Geometry: final body of the model. Coordinates: model frame, mm. Face numbers are marked on the shaded views. A direction names the side the tool comes from. Coordinates: 2 decimals unless noted, no trailing zeros. Order: outer loops, then holes, each group sorted by start corner. A loop starts at its lowest first (then second) coordinate and runs counter-clockwise, first axis right, second up. Notation, with made-up numbers: M 68.5,42 L 95.5,42 A10 ccw 95.5,51 Z; hole C 12,66 d7. An arc over 180 degrees is marked long. One line per question, with ' | ' between items.
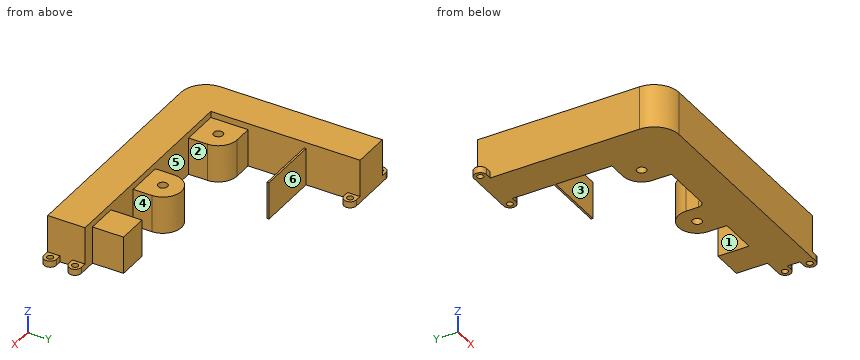
from build123d import *

# Parameters (mm, degrees)
F1_DEPTH = 70
F0_R     = 7.5
F0_W     = 100
F0_H     = 3
F0_W_2   = 50
F0_H_2   = 50
F2_DEPTH = 60
F0_R_2   = 5
F3_DEPTH = 10


with BuildPart() as f1:
    # F0 (on Top) → F1 (new body)
    with BuildSketch(Plane.XY):
        with BuildLine():
            Line((0, 280), (0, 40))
            ThreePointArc((0, 40), (11.715729, 11.715729), (40, 0))
            Line((40, 0), (400, 0))
            Line((400, 0), (400, 20))
            Line((400, 20), (400, 40))
            Line((400, 40), (400, 60))
            Line((400, 60), (380, 60))
            Line((380, 60), (330, 60))
            Line((330, 60), (270, 60))
            Line((270, 60), (210, 60))
            Line((210, 60), (200, 60))
            Line((200, 60), (120, 60))
            Line((120, 60), (60, 60))
            Line((60, 60), (60, 120))
            Line((60, 120), (60, 210))
            Line((60, 210), (60, 213))
            Line((60, 213), (60, 280))
            Line((60, 280), (60, 300))
            Line((60, 300), (0, 300))
            Line((0, 300), (0, 280))
        make_face()
    extrude(amount=F1_DEPTH)

    # F0 (on Top) → F2 (join)
    with BuildSketch(Plane.XY):
        with BuildLine():
            Line((90, 120), (60, 120))
            Line((60, 120), (60, 60))
            Line((60, 60), (120, 60))
            Line((120, 60), (120, 90))
            ThreePointArc((120, 90), (111.213203, 111.213203), (90, 120))
        make_face()
        with Locations((90, 90)):
            Circle(F0_R, mode=Mode.SUBTRACT)
        with BuildLine():
            Line((210, 60), (270, 60))
            Line((270, 60), (270, 90))
            ThreePointArc((270, 90), (240, 120), (210, 90))
            Line((210, 90), (210, 70))
            Line((210, 70), (210, 60))
        make_face()
        with Locations((240, 90)):
            Circle(F0_R, mode=Mode.SUBTRACT)
        with Locations((110, 211.5)):
            Rectangle(F0_W, F0_H)
        with Locations((355, 85)):
            Rectangle(F0_W_2, F0_H_2)
    extrude(amount=F2_DEPTH)

    # F0 (on Top) → F3 (join)
    with BuildSketch(Plane.XY):
        with BuildLine():
            Line((200, 60), (210, 60))
            Line((210, 60), (210, 70))
            ThreePointArc((210, 70), (207.071068, 62.928932), (200, 60))
        make_face()
        with BuildLine():
            Line((400, 60), (400, 40))
            Line((400, 40), (410, 40))
            ThreePointArc((410, 40), (420, 50), (410, 60))
            Line((410, 60), (400, 60))
        make_face()
        with Locations((410, 50)):
            Circle(F0_R_2, mode=Mode.SUBTRACT)
        with BuildLine():
            Line((400, 20), (400, 0))
            Line((400, 0), (410, 0))
            ThreePointArc((410, 0), (420, 10), (410, 20))
            Line((410, 20), (400, 20))
        make_face()
        with Locations((410, 10)):
            Circle(F0_R_2, mode=Mode.SUBTRACT)
        with BuildLine():
            Line((70, 300), (60, 300))
            Line((60, 300), (60, 280))
            Line((60, 280), (70, 280))
            ThreePointArc((70, 280), (80, 290), (70, 300))
        make_face()
        with Locations((70, 290)):
            Circle(F0_R_2, mode=Mode.SUBTRACT)
        with BuildLine():
            Line((-10, 280), (0, 280))
            Line((0, 280), (0, 300))
            Line((0, 300), (-10, 300))
            ThreePointArc((-10, 300), (-20, 290), (-10, 280))
        make_face()
        with Locations((-10, 290)):
            Circle(F0_R_2, mode=Mode.SUBTRACT)
    extrude(amount=F3_DEPTH)


solid = f1.part
1. Draft query along X for the marked faces 4, 5 and 6. Return one class per face: pulls with the +X half, pulls with the -X half, needs draft (parallel to the pull), parting line crosses it, or undercut.
Response values:
face 4: undercut | face 5: undercut | face 6: needs draft
2. Material intervals for line 1 (Y direction, x = 410, z = 3); line 2 (Y direction, x = 90, z = 19.5); line 3 (X direction, y = 77.5, z = 22.5), sorted ascending. Write a range as [from, to].
Response values:
line 1: y = [0, 5], [15, 20], [40, 45], [55, 60] | line 2: y = [0, 82.5], [97.5, 120], [210, 213] | line 3: x = [0, 120], [210, 270], [330, 380]
3. Pin query (flat end, axial travel): P1, Ø1, axis at y = 83, z = 20.5, coming from the +X side; P2, Ø10, axis at y = 209, z = 22.5, coming from the +X side; P3, Ø6, axis at x = 267, z = 47, coming from the +Y side. Return the tip coordinate at first contact, or that it passes through.
Response values:
P1: stops at x = 380 | P2: stops at x = 160 | P3: stops at y = 108
4. Section C-C, the plane y = 290. Output: boundary loops of the cut face in (x, z).
Response values:
outline: M -20,0 L -15,0 L -15,10 L -20,10 Z; M -5,0 L 65,0 L 65,10 L 60,10 L 60,70 L 0,70 L 0,10 L -5,10 Z; M 75,0 L 80,0 L 80,10 L 75,10 Z
5. Section D-D, the plane x = 360.5. Output: boundary loops of the cut face in (y, z), and give its area (3 significant figures).
Response values:
outline: M 0,0 L 110,0 L 110,60 L 60,60 L 60,70 L 0,70 Z | area: 7,200 mm^2
6. Section B-B, the plane z = 30.5. Output: boundary loops of the cut face in (x, y).
Response values:
outline: M 0,40 A40 ccw 40,0 L 400,0 L 400,60 L 380,60 L 380,110 L 330,110 L 330,60 L 270,60 L 270,90 A30 ccw 210,90 L 210,60 L 120,60 L 120,90 A30 ccw 90,120 L 60,120 L 60,210 L 160,210 L 160,213 L 60,213 L 60,300 L 0,300 Z; hole C 90,90 d15; hole C 240,90 d15
7. Access query for the marked faces 1, 2 and 3. Directions: +Z, -Z, +X, -X, +Y, -Y. A direction counts if a zero-diameter tool reaches every point of the face in a straight line with its end or side. Return the directions, or none.
Response values:
face 1: +Z, -Z, +Y | face 2: +Z, -Z | face 3: +Z, -Z, +X
8. Section A-A, the plane y = 50. Output: boundary loops of the cut face in (x, z).
Response values:
outline: M 0,0 L 405,0 L 405,10 L 400,10 L 400,70 L 0,70 Z; M 415,0 L 420,0 L 420,10 L 415,10 Z
